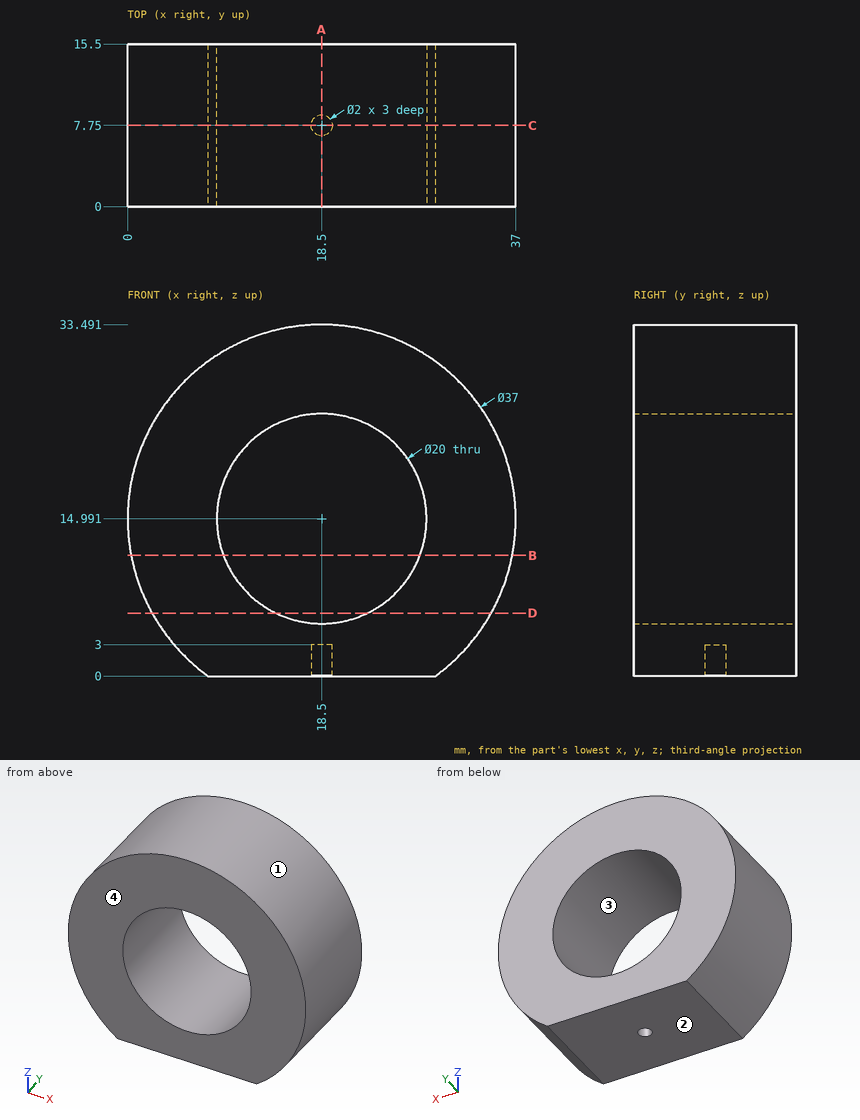
Job drawing, mm, ordinate dimensions from the low corner. One solid piece. Coordinates: 2 decimals unless noted, no trailing zeros. Order: outer loops, then holes, each group sorted by start corner. A loop starts at its lowest first (then second) coordinate and runs counter-clockwise, first axis right, second up. Notation, with made-up numbers: M 54.5,-29 L 93.5,-29 A8 cw 93.5,-15 Z; hole C 2.25,81 d11. An arc over 180 degrees is marked long. Answer as CSV lines item,"result".
(1) Wall check: line 1 along Y through (x, z) = (18.5, 0.85); line 2 along Z through (x, y) = (26.5, 8.5) (1 decimal); line 3 along X through (y, z) = (3.5, 9) (1 decimal). Give the ranges that are in metal, low to high.
Geometry says:
line 1,"y = 0 to 6.75, 8.75 to 15.5"
line 2,"z = 0 to 9, 21 to 31.7"
line 3,"x = 1 to 10.5, 26.5 to 36"
(2) Band-saw the part on B-B, the plane z = 11.5. List the corners of the cut face in (x, y).
Geometry says:
outline,"M 0.33,0 L 9.13,0 L 9.13,15.5 L 0.33,15.5 Z; M 27.87,0 L 36.67,0 L 36.67,15.5 L 27.87,15.5 Z"
(3) Pull direction Z, two halves, no side cores. Call the marked faces 1, 2, 3 and 4: +Z half, -Z half, draft (parallel to the pull), parting line (faces both ways), or undercut.
Geometry says:
face 1,"parting line"
face 2,"-Z half"
face 3,"undercut"
face 4,"draft"
(4) Band-saw the part on C-C, the plane y = 7.75. List the corners of the cut face in (x, z), then the cut area to 3 significant figures.
Geometry says:
outline,"M 7.66,0 L 17.5,0 L 17.5,3 L 19.5,3 L 19.5,0 L 29.34,0 A18.5 ccw long Z; hole C 18.5,14.99 d20"
area,"703 mm2"
(5) Flat gauge pins, fed straight in: pin 1 (2 mm diameter, centred on y = 6.5, z = 22.5, fed in from -X); pin 2 (5 mm diameter, centred on y = 2.5, z = 28, fed in from +X) (1 decimal); pin 3 (4 mm diameter, centred on y = 12, z = 9.5, fed in from +X); pin 4 (16 mm diameter, centred on x = 18.5, z = 14.99, fed in from +Y). Where does each tip first touch, or does it go through?
Geometry says:
pin 1,"stops at x = 1.18"
pin 2,"stops at x = 33.7"
pin 3,"stops at x = 36.67"
pin 4,"passes through"
(6) Band-saw the part on A-A, the plane x = 18.5. List the corners of the cut face in (y, z).
Geometry says:
outline,"M 0,0 L 6.75,0 L 6.75,3 L 8.75,3 L 8.75,0 L 15.5,0 L 15.5,4.99 L 0,4.99 Z; M 0,24.99 L 15.5,24.99 L 15.5,33.49 L 0,33.49 Z"
(7) Band-saw the part on D-D, the plane z = 6. List the corners of the cut face in (x, y).
Geometry says:
outline,"M 2.33,0 L 14.12,0 L 14.12,15.5 L 2.33,15.5 Z; M 22.88,0 L 34.67,0 L 34.67,15.5 L 22.88,15.5 Z"
